Input: part model. Units: mm. Frame: model coordinates. A direction names the side the tool comes from. Round coordinates to 2 decimals unless told otherwise and drop trailing zeros. Loops run counter-clockwise (first coordinate to the right, second up) from the corner with the lowest first, then second, coordinate; pieces in that order, holes last. Notation, with made-up numbers: M 74.25,39.5 L 132.25,39.5 A15 cw 132.25,60.5 Z; hole C 73.25,68.5 d10. An arc over 180 degrees is marked long. Use one line per item in the form item = value. Start each with the question number.
Q1. First-contact query: P1, Ø5, axis at x = -22.5, z = 0, coming from the +Y side; P2, Ø5, axis at x = -10, z = 14.5, coming from the -Y side; P3, Ø6, axis at y = 5.5, z = -21, coming from the +X side. Flat tips, straight axial feed; report the tip coordinate or a pass-through.
Q2. Section query D-D, the plane y = 13.5. Output: boundary loops of the cut face in (x, z).
Q3. Access query for faces 4 (the cylindrical face through (-24.503, 3.719, -0.631)), 5 (the flat face through (2, 16, 7)), 6 (the flat face through (0, 1.5, 12)), 7 (the cylindrical face through (-4.032, 17.014, -6.324)), 8 (the flat face through (0.1, 19, -4.4)). Directions: +Z, -Z, +X, -X, +Y, -Y. A direction counts if a zero-diameter tool reaches every point of the face in a straight line with its end or side. Return the directions, or none.
Q4. Mould query, pull axis X, two halves, no side actions, for faces 1 (the flat face through (0, 0, -5)), 2 (the flat face through (0, 10, -4)), 3 (the cylindrical face through (5.85, 3.27, 26.36)). Classes: pulls with the +X half, pulls with the -X half, needs draft (parallel to the pull), parting line crosses it, or undercut.
Q5. Section query B-B, the plane y = 7.25. Output: boundary loops of the cut face in (x, z).
Q6. Section query C-C, the plane z = 0. State how many separate pieces and enclosed holes the cut face has, and give its area (3 significant figures).
Q7. Ray query, line 1 along Y through (x, z) = (21, -10.5); line 2 along Z through (x, y) = (-11.25, 2.55); line 3 along Z through (x, y) = (-22.5, 4.25). Return the intervals inside material, ascending.
```python
from build123d import *

# Parameters (mm, degrees)
CUT_EXTRUDE_1_DEPTH = 43.649736224
HOLE_WIZARD_M5_1_D  = 4.2
CHAMFER_1_SIZE      = 2
CHAMFER_2_SIZE      = 1


with BuildPart() as part:
    # 草图1 → 旋转1 (revolve)
    with BuildSketch(Plane.XY, mode=Mode.PRIVATE) as revolve_1_sk:
        Polygon((0, 19), (0, 0), (10, 0), (10, 1.5), (27, 1.5), (27, 6), (9, 6), (9, 10), (7.5, 10), (7.5, 15), (6.8, 15), (6.8, 16), (7.5, 16), (7.5, 19), align=None)
    revolve(revolve_1_sk.sketch.rotate(Axis((0, 19, 0), (0, -1, 0)), 180), axis=Axis((0, 19, 0), (0, -1, 0)))

    # 草图2 → 切除-拉伸1 (cut, through all)
    with BuildSketch(Plane(origin=(0, 19, 0), x_dir=(1, 0, 0), z_dir=(0, 1, 0))):
        with BuildLine():
            Line((-3, 4), (3, 4))
            ThreePointArc((3, 4), (0, -5), (-3, 4))
        make_face()
    extrude(amount=-CUT_EXTRUDE_1_DEPTH, mode=Mode.SUBTRACT)

    # M5 螺纹孔1 (through all)
    with Locations(Plane(origin=(0, 6, 0), x_dir=(1, 0, 0), z_dir=(0, 1, 0))):
        with Locations((-11.25, 19.485571585), (11.25, 19.485571585), (22.5, 0), (11.25, -19.485571585), (-11.25, -19.485571585), (-22.5, 0)):
            Hole(HOLE_WIZARD_M5_1_D / 2)

    # 倒角1
    chamfer_1_edges = [part.edges().sort_by_distance(p)[0] for p in [
        (9, 6, 0),
    ]]
    chamfer(chamfer_1_edges, length=CHAMFER_1_SIZE)

    # 倒角2
    chamfer_2_edges = [part.edges().sort_by_distance(p)[0] for p in [
        (27, 6, 0),
        (7.5, 19, 0),
    ]]
    chamfer(chamfer_2_edges, length=CHAMFER_2_SIZE)


solid = part.part
```
Results found:
q1.P1 = 6
q1.P2 = 1.5
q1.P3 = 20.09
q2.outline = C 0,0 d15; hole M -3,-4 L 3,-4 A5 ccw long Z
q3.face_4 = +Y, -Y
q3.face_5 = none
q3.face_6 = -Y
q3.face_7 = +Y
q3.face_8 = +Z, -Z, +X, -X, +Y
q4.face_1 = needs draft
q4.face_2 = undercut
q4.face_3 = parting line crosses it
q5.outline = C 0,0 d19.5; hole M -3,-4 L 3,-4 A5 ccw long Z
q6.separate_pieces = 4
q6.enclosed_holes = 0
q6.area = 253 mm²
q7.line_1 = 1.5 to 6
q7.line_2 = -24.54 to -21.59, -17.39 to 17.39, 21.59 to 24.54
q7.line_3 = -14.92 to -2.1, 2.1 to 14.92
